from build123d import *

# Parameters (mm, degrees)
ESBO_O1_R                = 20
RESSALTO_EXTRUS_O1_DEPTH = 5
ESBO_O2_R                = 5
CORTE_EXTRUS_O2_DEPTH    = 5
FILETE3_R                = 2


with BuildPart() as part:
    # Esboço1 → Ressalto-extrusão1 (new, symmetric)
    with BuildSketch(Plane.XY):
        Circle(ESBO_O1_R)
    extrude(amount=RESSALTO_EXTRUS_O1_DEPTH, both=True)

    # Esboço2 → Corte-extrusão2 (cut, symmetric)
    with BuildSketch(Plane.XY):
        Circle(ESBO_O2_R)
    extrude(amount=CORTE_EXTRUS_O2_DEPTH, both=True, mode=Mode.SUBTRACT)

    # Filete3
    filete3_edges = [part.edges().sort_by_distance(p)[0] for p in [
        (-20, 0, -5),
        (-20, 0, 5),
    ]]
    fillet(filete3_edges, radius=FILETE3_R)


solid = part.part
Check sheet for the modelled part. Datum: model origin and axes. Units: mm. Give positions to 0.01 mm unless a question says otherwise; leave off trailing zeros. Write each loop counter-clockwise with the first axis right and the second up, starting at its lowest first coordinate (ties: lowest second). Pieces come first, ordered by that corner, then holes. Notation, with made-up numbers: M 50.5,-16.75 L 66.5,-16.75 A32 cw 66.5,22.25 Z; hole C 10,22 d8. An arc over 180 degrees is marked long. Use one line per item in the form item = value.
(1) Section check A-A on y = 0. Record the boundary of the cut face in (x, z), plus the area to 3 significant figures.
Answer block:
outline = M -20,-3 A2 ccw -18,-5 L -5,-5 L -5,5 L -18,5 A2 ccw -20,3 Z; M 5,-5 L 18,-5 A2 ccw 20,-3 L 20,3 A2 ccw 18,5 L 5,5 Z
area = 297 mm2
(2) Section check C-C on z = -2.5. Record the boundary of the cut face in (x, y).
Answer block:
outline = C 0,0 d40; hole C 0,0 d10
(3) Depth check by flat-ended pin: P1, Ø3, axis at x = -1, z = -2, coming from the +Y side; P2, Ø1, axis at x = 4.5, z = -3.5, coming from the -Y side; P3, Ø6, axis at y = -12.5, z = -3, coming from the +X side. Enter the tip coordinate at first touch or a pass-through.
Answer block:
P1 = 20
P2 = -19.57
P3 = 17.6
(4) Draft check along X on faces 1 (the cylindrical face through (-4.336, -19.524, 0.042)), 2 (the flat face through (4, -4, 5)), 3 (the cylindrical face through (-1.08, -4.88, 0.07)). Enter one of: pulls with the +X half, pulls with the -X half, needs draft (parallel to the pull), parting line crosses it, or undercut.
Answer block:
face_1 = parting line crosses it
face_2 = needs draft
face_3 = undercut
(5) Material ranges on line 1 along Y through (x, z) = (0, 0.5); line 2 along X through (y, z) = (-2, -2.25); line 3 along Y through (x, z) = (-2, 4), recorded low to high.
Answer block:
line_1 = -20 to -5, 5 to 20
line_2 = -19.9 to -4.58, 4.58 to 19.9
line_3 = -19.63 to -4.58, 4.58 to 19.63
